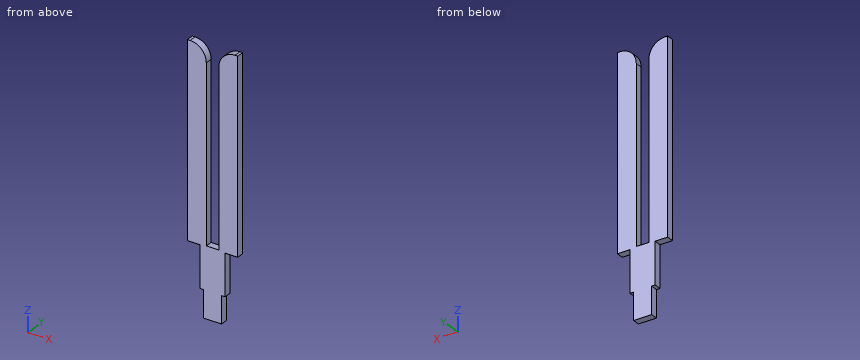
```python
from build123d import *

# Parameters (mm, degrees)
BOX017_W     = 2.8
BOX017_H     = 0.4
BOX017_DEPTH = 14.4
BOX018_W     = 0.7
BOX018_H     = 0.4
BOX018_DEPTH = 10.55
BOX019_W     = 0.7
BOX019_H     = 0.4
BOX019_DEPTH = 3.8
BOX020_W     = 0.7
BOX020_H     = 0.4
BOX020_DEPTH = 3.8
BOX021_W     = 0.2
BOX021_H     = 0.4
BOX021_DEPTH = 1.5
BOX022_W     = 0.2
BOX022_H     = 0.4
BOX022_DEPTH = 1.5
FILLET003_R  = 0.9


with BuildPart() as part:
    # Box017 → Box017 (join)
    with BuildSketch(Plane(origin=(-20.85, -2.74, -1.5), x_dir=(1, 0, 0), z_dir=(0, 0, 1))):
        with Locations((1.4, 0.2)):
            Rectangle(BOX017_W, BOX017_H)
    extrude(amount=BOX017_DEPTH)

    # Box018 → Box018 (cut)
    with BuildSketch(Plane(origin=(-19.8, -2.74, 2.35), x_dir=(1, 0, 0), z_dir=(0, 0, 1))):
        with Locations((0.35, 0.2)):
            Rectangle(BOX018_W, BOX018_H)
    extrude(amount=BOX018_DEPTH, mode=Mode.SUBTRACT)

    # Box019 → Box019 (cut)
    with BuildSketch(Plane(origin=(-20.85, -2.74, -1.5), x_dir=(1, 0, 0), z_dir=(0, 0, 1))):
        with Locations((0.35, 0.2)):
            Rectangle(BOX019_W, BOX019_H)
    extrude(amount=BOX019_DEPTH, mode=Mode.SUBTRACT)

    # Box020 → Box020 (cut)
    with BuildSketch(Plane(origin=(-18.75, -2.74, -1.5), x_dir=(1, 0, 0), z_dir=(0, 0, 1))):
        with Locations((0.35, 0.2)):
            Rectangle(BOX020_W, BOX020_H)
    extrude(amount=BOX020_DEPTH, mode=Mode.SUBTRACT)

    # Box021 → Box021 (cut)
    with BuildSketch(Plane(origin=(-20.15, -2.74, -1.5), x_dir=(1, 0, 0), z_dir=(0, 0, 1))):
        with Locations((0.1, 0.2)):
            Rectangle(BOX021_W, BOX021_H)
    extrude(amount=BOX021_DEPTH, mode=Mode.SUBTRACT)

    # Box022 → Box022 (cut)
    with BuildSketch(Plane(origin=(-18.95, -2.74, -1.5), x_dir=(1, 0, 0), z_dir=(0, 0, 1))):
        with Locations((0.1, 0.2)):
            Rectangle(BOX022_W, BOX022_H)
    extrude(amount=BOX022_DEPTH, mode=Mode.SUBTRACT)

    # Fillet003
    fillet003_edges = [part.edges().sort_by_distance(p)[0] for p in [
        (-19.8, -2.54, 12.9),
        (-19.1, -2.54, 12.9),
    ]]
    fillet(fillet003_edges, radius=FILLET003_R)


with BuildPart() as part_1:
    # Body003 placement: moved
    add(part.part.moved(Location((2.38, 5.0875, 0))))


solid = part_1.part
```
Source: CAD feature listing. Evaluate the final solid. Frame: model axes, mm. Round coordinates to 2 decimals unless told otherwise and drop trailing zeros. Loops run counter-clockwise (first coordinate to the right, second up) from the corner with the lowest first, then second, coordinate; pieces in that order, holes last.
1. Section query B-B on y = 2.65. Output: boundary loops of the cut face in (x, z).
2. Section query D-D on z = 1.25. Output: boundary loops of the cut face in (x, y), and give its area (3 significant figures).
3. Section query A-A on z = 3. Output: boundary loops of the cut face in (x, y), and give its area (3 significant figures).
4. Ray query, L1, parallel to X at y = 2.55, z = 6.25; L2, parallel to X at y = 2.5, z = 2; L3, parallel to Z at x = -16.9, y = 2.6. Return the intervals inside material, ascending.
5. Section query C-C on x = -17.15. Output: boundary loops of the cut face in (y, z), and give its area (3 significant figures).
Answers below:
1. outline: (-18.47, 2.3) - (-17.77, 2.3) - (-17.77, 0) - (-17.57, 0) - (-17.57, -1.5) - (-16.57, -1.5) - (-16.57, 0) - (-16.37, 0) - (-16.37, 2.3) - (-15.67, 2.3) - (-15.67, 12.9) - (-15.82, 12.9) arc R0.9 ccw to (-16.72, 12) - (-16.72, 2.35) - (-17.42, 2.35) - (-17.42, 12) arc R0.9 ccw to (-18.32, 12.9) - (-18.47, 12.9) - close
2. outline: (-17.77, 2.35) - (-16.37, 2.35) - (-16.37, 2.75) - (-17.77, 2.75) - close
2. area: 0.560 mm2
3. outline: (-18.47, 2.35) - (-17.42, 2.35) - (-17.42, 2.75) - (-18.47, 2.75) - close; (-16.72, 2.35) - (-15.67, 2.35) - (-15.67, 2.75) - (-16.72, 2.75) - close
3. area: 0.840 mm2
4. L1: x = -18.47 to -17.42, -16.72 to -15.67
4. L2: x = -17.77 to -16.37
4. L3: z = -1.5 to 2.35
5. outline: (2.35, -1.5) - (2.75, -1.5) - (2.75, 2.35) - (2.35, 2.35) - close
5. area: 1.54 mm2
